Autodesk Inventor part; units mm, degrees
ref_plane "YZ Plane" through (0, 0, 0) normal (1, 0, 0) x (0, 1, 0)
ref_plane "XZ Plane" through (0, 0, 0) normal (0, 1, 0) x (-1, 0, 0)
ref_plane "XY Plane" through (0, 0, 0) normal (0, 0, 1) x (1, 0, 0)
sketch "Skizze1" plane through (0, 0, 0) normal (1, 0, 0) x (0, 1, 0)
  circle A0 centre (0, 0) radius 10
  line L0 (15, 0) -> (15, -40)
  line L1 (15, -40) -> (-15, -40)
  line L2 (-15, -40) -> (-15, 0)
  line L3 (15, 0) -> (15, 20)
  line L4 (15, 20) -> (-15, 20)
  line L5 (-15, 20) -> (-15, 0)
  dimension "d0" = 20
  dimension "d2" = 40
  dimension "d3" = 30
  dimension "d4" = 90
  dimension "d40" = 20
extrude "Extrusion1" add sketch "Skizze1" along normal blind 30
sketch "Skizze3" plane through (30, 0, 0) normal (1, 0, 0) x (0, 0, -1)
  line L0 (0, 0) -> (-20, 0)
  line L1 (-20, 0) -> (-20, 3)
  line L2 (-20, 3) -> (0, 3)
  line L3 (0, 3) -> (0, 0)
  line L4 (0, 0) -> (-20, 0)
  line L5 (-20, 0) -> (-20, -3)
  line L6 (-20, -3) -> (0, -3)
  line L7 (0, -3) -> (0, 0)
  dimension "d7" = 20
  dimension "d8" = 3
  dimension "d9" = 3
extrude "Extrusion2" cut sketch "Skizze3" against normal through all
sketch "Skizze6" plane through (0, 0, 0) normal (-1, 0, 0) x (0, 0, 1)
  arc A0 (9.5394, 3) -> (9.5394, -3) centre (0, 0) ccw
  line L0 (0, 0) -> (-30, 0)
  dimension "d31" = 30
hole "Bohrung3" at (0, 0, -30) direction (1, 0, 0) diameter 4.134 end through all
fillet "Rundung1" radius 5 2 edges at (0, 0, -40) (30, 0, -40)
sketch "Skizze9" plane through (0, 15, 20) normal (0, 1, 0) x (1, 0, 0)
  line L0 (30, 47.933) -> (0, 47.933)
  line L1 (5, 60) -> (25, 60)
  line L2 (15, 60) -> (15, 48)
  circle A0 centre (15, 48) radius 10
  point P0 (0, 20)
  dimension "d79" = 12
  dimension "d80" = 20
extrude "Extrusion4" cut sketch "Skizze9" against normal through all
sketch "Skizze10" plane through (0, 15, 20) normal (0, 1, 0) x (1, 0, 0)
  line L0 (0, 0) -> (30, 0)
  line L1 (15, 0) -> (15, 5)
  point P0 (0, 20)
  dimension "d55" = 5
hole "Bohrung5" at (15, 15, 15) direction (0, -1, 0) diameter 5.2 depth 15 tip angle 118
sketch "Skizze12" plane through (0, -15, 20) normal (0, -1, 0) x (1, 0, 0)
  circle A0 centre (15, -5) radius 2.6
  line L0 (15, -5) -> (15, -13.3811)
  circle A1 centre (15, -5) radius 2.5
  point P0 (0, -20)
  dimension "d71" = 5
hole "Bohrung7" at (15, -15, 15) direction (0, 1, 0) diameter 4.134 end through all
properties part number "Verbindung" material "Edelstahl"
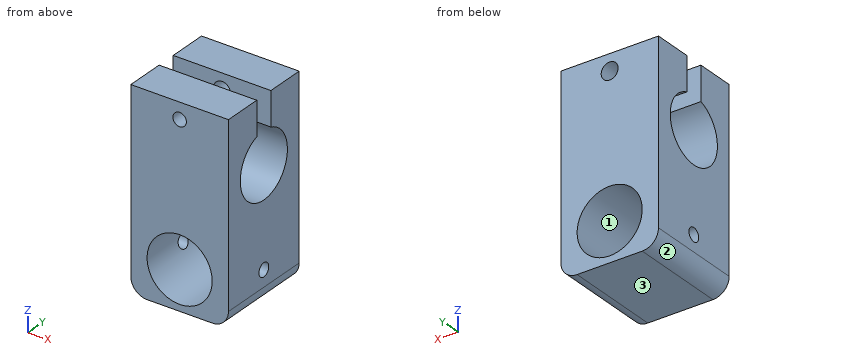
Design review of the part built by this model. Coordinates are the model's own, in mm. Face numbers are marked on the shaded views. Give positions to 0.01 mm unless a question says otherwise; leave off trailing zeros. Write each loop counter-clockwise with the first axis right and the second up, starting at its lowest first coordinate (ties: lowest second). Pieces come first, ordered by that corner, then holes. Notation, with made-up numbers: (-10.5, 9) - (30.5, 9) arc R31 cw to (30.5, 41) - close; hole circle Ø8 at (49.5, 2.25). An arc over 180 degrees is marked (long way). Return JSON: item names as keys, results as strings. Group by question number.
(1) We need section C-C, the plane x = 9. Give the boundary of the cut face in (y, z), then the cut area to 3 significant figures.
(2) To check wall thickness, follow probe 1 along Z at (x, y) = (15, 11); probe 2 along Y at (x, z) = (2, -30); probe 3 along X at (y, z) = (8, 15). State the ranges of each line that lie inside material, in increasing order.
(3) We need section B-B, the plane y = 13. Give the boundary of the cut face in (x, z).
(4) We need section A-A, the plane z = 0. Give the boundary of the cut face in (x, y).
(5) We need section D-D, the plane y = 6. Give the boundary of the cut face in (x, z).
(6) Mouldability with a two-part tool opening along X and no side actions: class the marked faces 1, 2 and 3 as +X half, -X half, draft (parallel to the pull), parting line (faces both ways), or undercut.
Reported:
{
 "1": {"outline": "(-15, -40) - (15, -40) - (15, -36) - (-15, -36) - close; (-15, -20) - (15, -20) - (15, 20) - (3, 20) - (3, 9.54) arc R10 cw (long way) to (-3, 9.54) - (-3, 20) - (-15, 20) - close", "area": "945 mm2"},
 "2": {"probe 1": "z = -40 to -38, -18 to 12.4, 17.6 to 20", "probe 2": "y = -15 to -2.07, 2.07 to 15", "probe 3": "x = 0 to 12.4, 17.6 to 30"},
 "3": {"outline": "(0, -35) arc R5 ccw to (5, -40) - (25, -40) arc R5 ccw to (30, -35) - (30, 20) - (0, 20) - close; hole circle Ø20 at (15, -28); hole circle Ø5.2 at (15, 15)"},
 "4": {"outline": "(0, -15) - (30, -15) - (30, -10) - (0, -10) - close; (0, 10) - (30, 10) - (30, 15) - (0, 15) - close"},
 "5": {"outline": "(0, -35) arc R5 ccw to (5, -40) - (25, -40) arc R5 ccw to (30, -35) - (30, -8) - (0, -8) - close; (0, 8) - (30, 8) - (30, 20) - (0, 20) - close; hole circle Ø20 at (15, -28); hole circle Ø5.2 at (15, 15)"},
 "6": {"face 1": "undercut", "face 2": "-X half", "face 3": "draft"}
}
